Could you check a few things on this model? Use its own coordinates, in mm. Face numbers are marked on the shaded views. A direction names the side the tool comes from. Coordinates: 2 decimals unless noted, no trailing zeros. Loops run counter-clockwise (first coordinate to the right, second up) from the corner with the lowest first, then second, coordinate; pieces in that order, holes last.
from build123d import *

# Parameters (mm, degrees)
SKETCH_1_R          = 5
EXTRUDE_1_DEPTH     = 4.5
CUT_EXTRUDE_1_DEPTH = 2.25
CHAMFER_1_SIZE      = 1
SKETCH_3_R          = 1.5
CUT_EXTRUDE_2_DEPTH = 16.625


with BuildPart() as part:
    # 草图1 → 凸台-拉伸1 (new, symmetric)
    with BuildSketch(Plane(origin=(0, 0, 0), x_dir=(1, 0, 0), z_dir=(0, 1, 0))):
        with BuildLine():
            Line((0, 9), (-9.33664655, 9))
            ThreePointArc((-9.33664655, 9), (-19.626561658, 10.819906901), (-28.668030932, 16.058823529))
            ThreePointArc((-28.668030932, 16.058823529), (-34.997059424, 19.726065169), (-42.2, 21))
            Line((-42.2, 21), (-42.2, 12.5))
            ThreePointArc((-42.2, 12.5), (-29.7, 0), (-42.2, -12.5))
            Line((-42.2, -12.5), (-42.2, -21))
            ThreePointArc((-42.2, -21), (-34.997059424, -19.726065169), (-28.668030932, -16.058823529))
            ThreePointArc((-28.668030932, -16.058823529), (-19.626561658, -10.819906901), (-9.33664655, -9))
            Line((-9.33664655, -9), (0, -9))
            ThreePointArc((0, -9), (9, 0), (0, 9))
        make_face()
        with Locations(Location((0, 0, 0), (0, 0, 270))):
            Circle(SKETCH_1_R, mode=Mode.SUBTRACT)
    extrude(amount=EXTRUDE_1_DEPTH, both=True)

    # 草图2 → 切除-拉伸1 (cut)
    with BuildSketch(Plane(origin=(0, 4.5, 0), x_dir=(1, 0, 0), z_dir=(0, 1, 0))):
        with BuildLine():
            Line((-42.2, -12.5), (-42.2, -21))
            ThreePointArc((-42.2, -21), (-21.2, 0), (-42.2, 21))
            Line((-42.2, 21), (-42.2, 12.5))
            ThreePointArc((-42.2, 12.5), (-29.7, 0), (-42.2, -12.5))
        make_face()
    cut_extrude_1 = extrude(amount=-CUT_EXTRUDE_1_DEPTH, mode=Mode.SUBTRACT)

    # 镜向1: 切除-拉伸1 across plane
    add(cut_extrude_1.mirror(Plane.ZX), mode=Mode.SUBTRACT)

    # 倒角1
    chamfer_1_edges = [part.edges().sort_by_distance(p)[0] for p in [
        (-29.7, 2.25, 0),
        (-29.7, -2.25, 0),
    ]]
    chamfer(chamfer_1_edges, length=CHAMFER_1_SIZE)

    # 草图3 → 切除-拉伸2 (cut, symmetric)
    with BuildSketch(Plane.XY):
        with Locations(Location((0, 0, 0), (0, 0, 89.999999982))):
            Circle(SKETCH_3_R)
    extrude(amount=CUT_EXTRUDE_2_DEPTH, both=True, mode=Mode.SUBTRACT)


solid = part.part
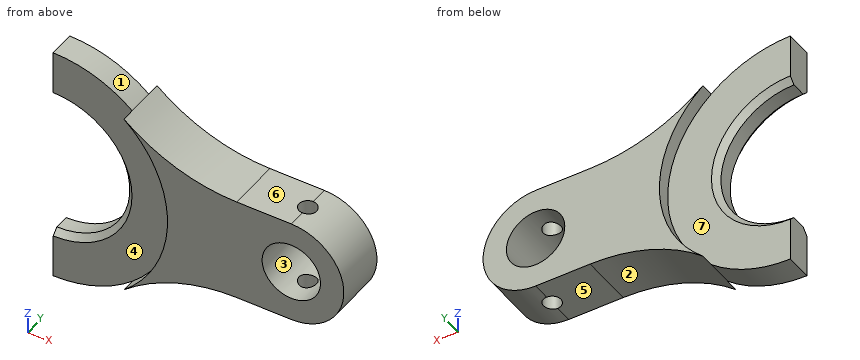
(1) I need wall thicknesses on probe 1 along Z at (x, y) = (0, -1.75); probe 2 along X at (y, z) = (-0.25, 0); probe 3 along Z at (x, y) = (-7, 1). Which ranges of each line are inside material? Lowest first, please.
Answers:
probe 1: z = -9 to -5, 5 to 9
probe 2: x = -29.7 to -5, 5 to 9
probe 3: z = -9 to 9
(2) Imagine slicing it at A-A, the plane y = 3.25. Write out the boundary of the cut face in (x, z).
Answers:
outline: (-28.67, -16.06) arc R30 cw to (-9.34, -9) - (0, -9) arc R9 ccw to (0, 9) - (-9.34, 9) arc R30 cw to (-28.67, 16.06) arc R21 cw to start; hole circle Ø10 at (0, 0)
(3) For pin 1 (2 mm diameter, centred on x = -30, y = -2, fed in from -Z); pin 2 (2 mm diameter, centred on x = -37, z = 11.5, fed in from +Y); pin 3 (3.5 mm diameter, centred on x = 0, y = 0, fed in from -Z), each with a flat end and sliding along its axis, tell me the tip position at first contact or that it passes through.
Answers:
pin 1: stops at z = -17.76
pin 2: stops at y = 2.25
pin 3: stops at z = -9
(4) Which directions (+Z, -Z, +X, -X, +Y, -Y) give clear straight access to the entire face, cutting with the end or side of a thin tool? Please do the marked faces 4, 5, 6 and 7.
Answers:
face 4: -X, -Y
face 5: -Z, +X, +Y, -Y
face 6: +Z, +X, +Y, -Y
face 7: -X, +Y
(5) Imagine slicing it at D-D, the plane x = 4. Write out the boundary of the cut face in (y, z).
Answers:
outline: (-4.5, -8.06) - (4.5, -8.06) - (4.5, -3) - (-4.5, -3) - close; (-4.5, 3) - (4.5, 3) - (4.5, 8.06) - (-4.5, 8.06) - close
(6) Imagine slicing it at C-C, the plane y = -0.25. Write out the boundary of the cut face in (x, z), and give its area (3 significant figures).
Answers:
outline: (-42.2, -21) arc R21 ccw to (-28.67, -16.06) arc R30 cw to (-9.34, -9) - (-1.48, -9) - (-1.48, -4.78) arc R5 cw to (-1.48, 4.78) - (-1.48, 9) - (-9.34, 9) arc R30 cw to (-28.67, 16.06) arc R21 ccw to (-42.2, 21) - (-42.2, 12.5) arc R12.5 cw to (-42.2, -12.5) - close; (1.48, -8.88) arc R9 ccw to (1.48, 8.88) - (1.48, 4.78) arc R5 cw to (1.48, -4.78) - close
area: 908 mm2
(7) Imagine slicing it at B-B, the plane z = 0. Write out the boundary of the cut face in (x, y), and give its area (3 significant figures).
Answers:
outline: (-29.7, -1.25) - (-28.7, -2.25) - (-21.2, -2.25) - (-21.2, -4.5) - (-5, -4.5) - (-5, 4.5) - (-21.2, 4.5) - (-21.2, 2.25) - (-28.7, 2.25) - (-29.7, 1.25) - close; (5, -4.5) - (9, -4.5) - (9, 4.5) - (5, 4.5) - close
area: 219 mm2
(8) We'd pull the mould along Z, two halves only. Please class the marked faces 1, 2 and 3: +Z half, -Z half, draft (parallel to the pull), parting line (faces both ways), or undercut.
Answers:
face 1: +Z half
face 2: -Z half
face 3: undercut
